```python
from build123d import *

# Parameters (mm, degrees)
F0_R     = 1.75
F1_DEPTH = 1.75
F2_DEPTH = 1.75


with BuildPart() as f1:
    # F0 (on Front) → F1 (new body)
    with BuildSketch(Plane.XZ):
        Polygon((17.5, 8.6541427299), (-17.5, 8.6541427299), (-17.5, -1.3458572701), (-12.5, -1.3458572701), (12.5, -1.3458572701), (17.5, -1.3458572701), align=None)
        with BuildLine():
            ThreePointArc((-10.75, 3.6541427299), (-11.2625631329, 2.4167058629), (-12.5, 1.9041427299))
            ThreePointArc((-12.5, 1.9041427299), (-13.7374368671, 4.891579597), (-10.75, 3.6541427299))
        make_face(mode=Mode.SUBTRACT)
        with Locations((0, 3.6541427299)):
            Circle(F0_R, mode=Mode.SUBTRACT)
        with BuildLine():
            ThreePointArc((14.25, 3.6541427299), (13.7374368671, 2.4167058629), (12.5, 1.9041427299))
            ThreePointArc((12.5, 1.9041427299), (11.2625631329, 2.4167058629), (10.75, 3.6541427299))
            ThreePointArc((10.75, 3.6541427299), (12.5, 5.4041427299), (14.25, 3.6541427299))
        make_face(mode=Mode.SUBTRACT)
    extrude(amount=F1_DEPTH)

    # F2 (add): a face of the model
    f2_faces = [f1.faces().sort_by_distance(p)[0] for p in [
        (17.1359945055, -1.75, 3.6541427299),
    ]]
    extrude(f2_faces, amount=-F2_DEPTH)


solid = f1.part
```
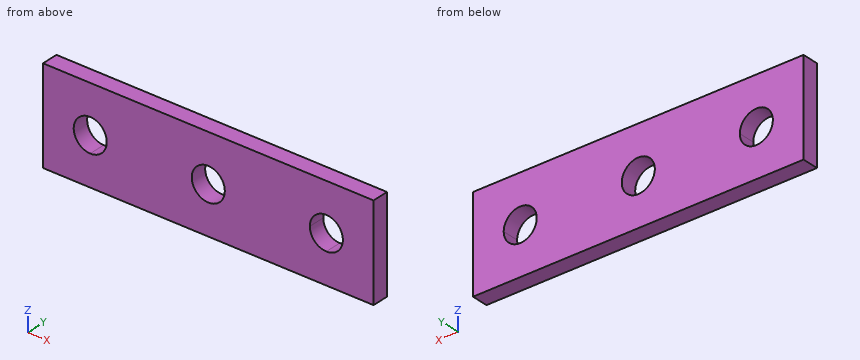
Check sheet for the modelled part. Datum: model origin and axes. Units: mm. Coordinates: 2 decimals unless noted, no trailing zeros. Write each loop counter-clockwise with the first axis right and the second up, starting at its lowest first coordinate (ties: lowest second). Pieces come first, ordered by that corner, then holes. Notation, with made-up numbers: (17, 72) - (39, 72) arc R11 cw to (39, 85) - close; hole circle Ø4 at (-32, -14). An arc over 180 degrees is marked (long way). One line per question, with ' | ' between items.
Item 1: Sectioned sample at A-A on y = -0.35. Record the boundary of the cut face in (x, z).
Determined:
outline: (-17.5, -1.35) - (17.5, -1.35) - (17.5, 8.65) - (-17.5, 8.65) - close; hole circle Ø3.5 at (-12.5, 3.65); hole circle Ø3.5 at (0, 3.65); hole circle Ø3.5 at (12.5, 3.65)
Item 2: Gauge pin test, flat end, axial feed: P1, Ø3, axis at x = 0, z = 3.65, coming from the +Y side. Record the tip position at first contact, or that the pin passes through.
Determined:
P1: passes through
Item 3: Sectioned sample at D-D on z = 4.25. Record the boundary of the cut face in (x, y), plus the area to 3 significant figures.
Determined:
outline: (-17.5, -1.75) - (-14.15, -1.75) - (-14.15, 0) - (-17.5, 0) - close; (-10.85, -1.75) - (-1.65, -1.75) - (-1.65, 0) - (-10.85, 0) - close; (1.65, -1.75) - (10.85, -1.75) - (10.85, 0) - (1.65, 0) - close; (14.15, -1.75) - (17.5, -1.75) - (17.5, 0) - (14.15, 0) - close | area: 44.0 mm2
Item 4: Sectioned sample at C-C on z = 2.5. Record the boundary of the cut face in (x, y), plus the area to 3 significant figures.
Determined:
outline: (-17.5, -1.75) - (-13.82, -1.75) - (-13.82, 0) - (-17.5, 0) - close; (-11.18, -1.75) - (-1.32, -1.75) - (-1.32, 0) - (-11.18, 0) - close; (1.32, -1.75) - (11.18, -1.75) - (11.18, 0) - (1.32, 0) - close; (13.82, -1.75) - (17.5, -1.75) - (17.5, 0) - (13.82, 0) - close | area: 47.4 mm2
Item 5: Sectioned sample at B-B on x = 0. Record the boundary of the cut face in (y, z), plus the area to 3 significant figures.
Determined:
outline: (-1.75, -1.35) - (0, -1.35) - (0, 1.9) - (-1.75, 1.9) - close; (-1.75, 5.4) - (0, 5.4) - (0, 8.65) - (-1.75, 8.65) - close | area: 11.4 mm2
Item 6: Thickness scan on line 1 (X direction, y = -0.25, z = 3.75); line 2 (Z direction, x = 0, y = -0.55); line 3 (X direction, y = -0.85, z = 2.5). Record the ranges inside material, lowest first. Write a range as [from, to].
Determined:
line 1: x = [-17.5, -14.25], [-10.75, -1.75], [1.75, 10.75], [14.25, 17.5] | line 2: z = [-1.35, 1.9], [5.4, 8.65] | line 3: x = [-17.5, -13.82], [-11.18, -1.32], [1.32, 11.18], [13.82, 17.5]
